Drawing for the job (mm, zero at the part's lowest x, y, z). Round coordinates to 2 decimals unless told otherwise and drop trailing zeros. Order: outer loops, then holes, each group sorted by start corner. A loop starts at its lowest first (then second) coordinate and runs counter-clockwise, first axis right, second up. Notation, with made-up numbers: (61, 33) -> (90, 33) arc R22 ccw to (90, 47) -> close; hole circle Ø3 at (-13, -5.5). An arc over 180 degrees is marked (long way). Use CSV: the item, a comma, the result in double quotes.
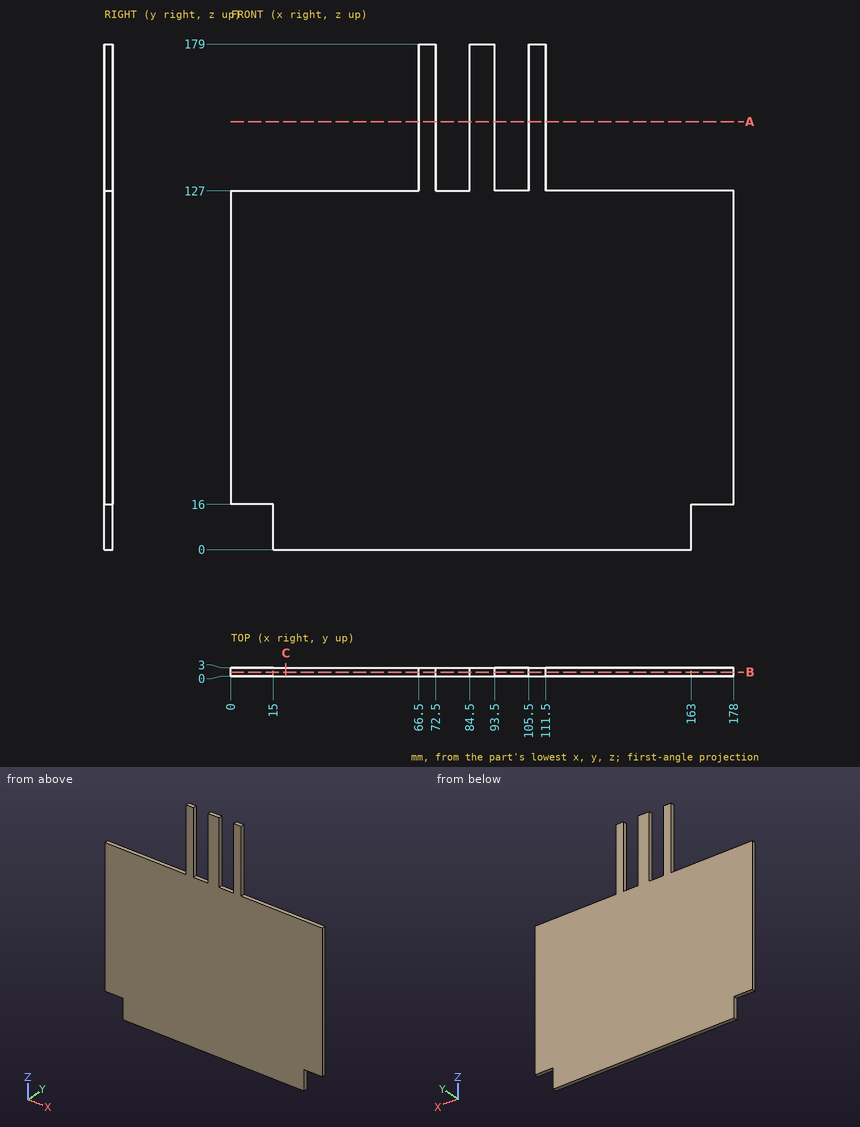
Q1. Cut at B-B (y = 1.4). Give the cut face in (x, z).
From the geometry:
outline,"(0, 16) -> (15, 16) -> (15, 0) -> (163, 0) -> (163, 16) -> (178, 16) -> (178, 127) -> (111.5, 127) -> (111.5, 179) -> (105.5, 179) -> (105.5, 127) -> (93.5, 127) -> (93.5, 179) -> (84.5, 179) -> (84.5, 127) -> (72.5, 127) -> (72.5, 179) -> (66.5, 179) -> (66.5, 127) -> (0, 127) -> close"
Q2. Cut at A-A (z = 151.5). Give the cut face in (x, y).
From the geometry:
outline,"(66.5, 0) -> (72.5, 0) -> (72.5, 3) -> (66.5, 3) -> close; (84.5, 0) -> (93.5, 0) -> (93.5, 3) -> (84.5, 3) -> close; (105.5, 0) -> (111.5, 0) -> (111.5, 3) -> (105.5, 3) -> close"
Q3. Probe line 1 along X through (y, z) = (0.4, 139.5); line 2 along Z through (x, y) = (143, 1.1); line 3 along X through (y, z) = (2.2, 13.5). List the from-to ranges inside material, lowest first.
From the geometry:
line 1,"x = 66.5 to 72.5, 84.5 to 93.5, 105.5 to 111.5"
line 2,"z = 0 to 127"
line 3,"x = 15 to 163"
Q4. Pin check, flat tips, straight feed: pin 1 (0.9 mm diameter, centred on x = 29.5, y = 2, fed in from +Z); pin 2 (0.9 mm diameter, centred on y = 2, z = 153.5, fed in from -X); pin 3 (0.9 mm diameter, centred on x = 172, y = 1, fed in from -Z). Stop position of each tip, or through.
From the geometry:
pin 1,"stops at z = 127"
pin 2,"stops at x = 66.5"
pin 3,"stops at z = 16"
Q5. Cut at C-C (x = 19.5). Give the cut face in (y, z).
From the geometry:
outline,"(0, 0) -> (3, 0) -> (3, 127) -> (0, 127) -> close"
